Could you check a few things on this model? Use its own coordinates, in mm. A direction names the side the tool comes from. Give positions to 0.01 mm unless a question says otherwise; leave off trailing zeros. Loops run counter-clockwise (first coordinate to the right, second up) from the corner with the lowest first, then second, coordinate; pieces in that order, holes last.
1. Imagine slicing it at B-B (x = -19). List the corners of the cut face in (y, z) for me, plus the area to 3 significant figures.
2. Imagine slicing it at C-C (z = -281). List the corners of the cut face in (x, y) for me, plus the area to 3 significant figures.
3. Thinking about a two-plate mould opening in Y: for faces 3 (the flat face through (-45, -1, 16)), 4 (the flat face through (-1, -50, 14)), 5 (the flat face through (-50, -1, 16)), which applies, +Y half, -Y half, draft (parallel to the pull), parting line (faces both ways), or undercut?
4. Imagine slicing it at A-A (y = -5). List the corners of the cut face in (x, z) for me.
5. I need wall thicknesses on line 1 along Y through (x, z) = (-7.5, -172); line 2 along Z through (x, y) = (46, -4). Which ranges of each line are inside material? Lowest first, please.
6. For faces 1 (the flat face through (-1, 50, 16)), 2 (the flat face through (-1, 45, 16)), which set-ups out of +Z, -Z, +X, -X, +Y, -Y let a thin tool reach every point of the face, with its end or its side?
```python
from build123d import *

# Parameters (mm, degrees)
SKETCH1_W               = 100
SKETCH1_H               = 100
SKETCH1_W_2             = 90
SKETCH1_H_2             = 90
BOSS_EXTRUDE1_DEPTH     = 1125
CUT_EXTRUDE1_DEPTH      = 51
CUT_EXTRUDE1_DEPTH_BACK = 51


with BuildPart() as part:
    # Sketch1 → Boss-Extrude1 (new body, symmetric)
    with BuildSketch(Plane.XY):
        Rectangle(SKETCH1_W, SKETCH1_H)
        Rectangle(SKETCH1_W_2, SKETCH1_H_2, mode=Mode.SUBTRACT)
    extrude(amount=BOSS_EXTRUDE1_DEPTH, both=True)

    # Sketch4 → Cut-Extrude1 (cut, two sides)
    with BuildSketch(Plane(origin=(0, 0, 0), x_dir=(0, 0, -1), z_dir=(1, 0, 0))) as cut_extrude1_sk:
        Polygon((-1125, 50), (-1025, -50), (-1125, -50), align=None)
        Polygon((1125, 50), (1025, -50), (1125, -50), align=None)
    extrude(amount=CUT_EXTRUDE1_DEPTH, mode=Mode.SUBTRACT)
    extrude(cut_extrude1_sk.sketch, amount=-CUT_EXTRUDE1_DEPTH_BACK, mode=Mode.SUBTRACT)


solid = part.part
```
Derived:
1. outline: (-50, -1025) - (-45, -1030) - (-45, 1030) - (-50, 1025) - close; (45, -1120) - (50, -1125) - (50, 1125) - (45, 1120) - close
1. area: 21,500 mm2
2. outline: (-50, -50) - (50, -50) - (50, 50) - (-50, 50) - close; hole (-45, -45) - (45, -45) - (45, 45) - (-45, 45) - close
2. area: 1,900 mm2
3. face 3: undercut
3. face 4: -Y half
3. face 5: draft
4. outline: (-50, -1070) - (-45, -1070) - (-45, 1070) - (-50, 1070) - close; (45, -1070) - (50, -1070) - (50, 1070) - (45, 1070) - close
5. line 1: y = -50 to -45, 45 to 50
5. line 2: z = -1071 to 1071
6. face 1: +Z, -Z, +X, -X, +Y
6. face 2: +Z, -Z
